The figure shows three views and two pictorial views of one solid part (mm, origin at its lowest corner). Answer the questions. Round coordinates to 2 decimals unless told otherwise and drop trailing zeros. Order: outer loops, then holes, each group sorted by start corner. A loop starts at its lowest first (then second) coordinate and runs counter-clockwise, first axis right, second up. Notation, with made-up numbers: (82.5, 25.25) -> (94.5, 25.25) arc R25 cw to (94.5, 41.25) -> close; hole circle Ø6 at (72.5, 61.5). An arc over 180 degrees is marked (long way). One line per item, written item: value. Start each with the question number.
1. Section D-D (x = 5.75) is taken. Give the vertices of the cut face in (y, z).
2. Consider line 1 (Z direction, x = 15, y = 1.35); line 2 (Z direction, x = 18, y = 0.3); line 3 (X direction, y = 0.4, z = 23). Determine where each line is inside the solid, lowest interval first.
3. Section C-C (z = 6.5) is taken. Give the vertices of the cut face in (x, y), then the cut area to 3 significant figures.
4. Section B-B (y = 0.65) is taken. Give the vertices of the cut face in (x, z).
5. Section A-A (x = 15) is taken. Give the vertices of the cut face in (y, z).
6. The mould has two halves that part along Z. Classify the marked faces 1, 2 and 3: released by +Z, released by -Z, zero draft, split by the parting line, or undercut.
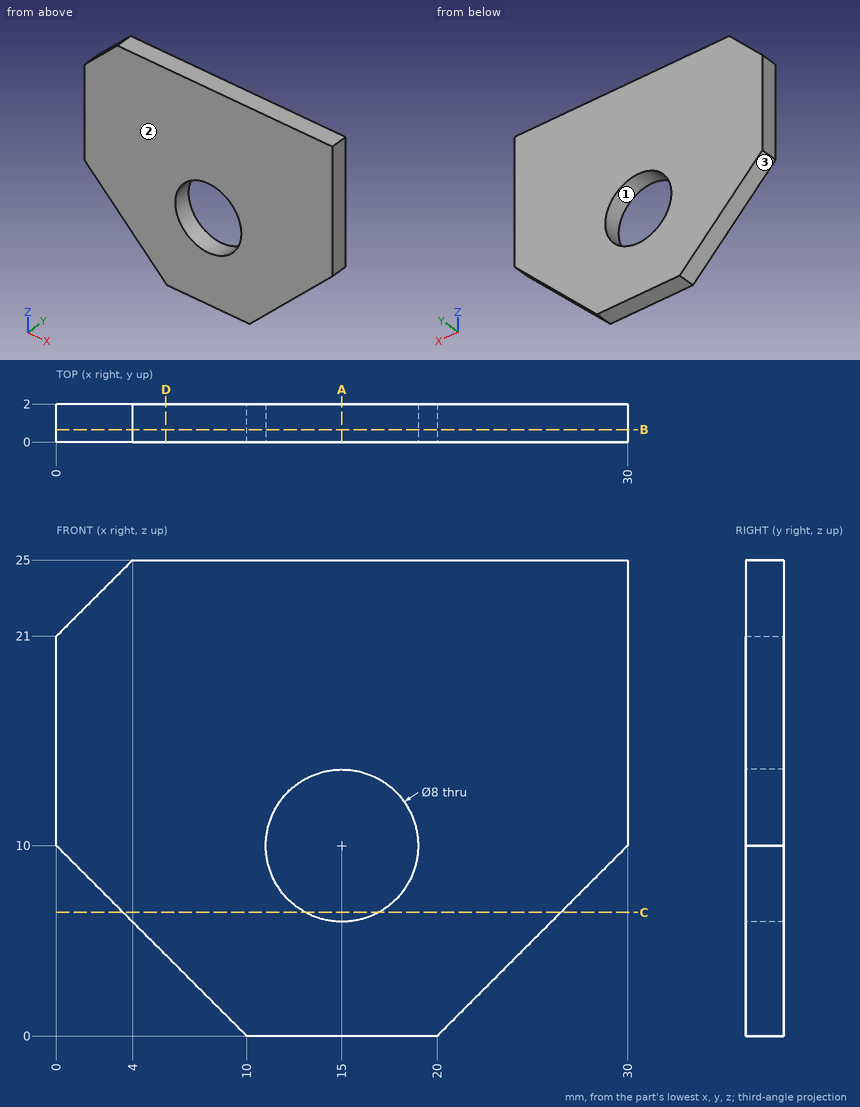
Answer:
1. outline: (0, 4.25) -> (2, 4.25) -> (2, 25) -> (0, 25) -> close
2. line 1: 0 to 6, 14 to 25
2. line 2: 0 to 7.35, 12.65 to 25
2. line 3: 2 to 30
3. outline: (3.5, 0) -> (13.06, 0) -> (13.06, 2) -> (3.5, 2) -> close; (16.94, 0) -> (26.5, 0) -> (26.5, 2) -> (16.94, 2) -> close
3. area: 38.3 mm^2
4. outline: (0, 10) -> (10, 0) -> (20, 0) -> (30, 10) -> (30, 25) -> (4, 25) -> (0, 21) -> close; hole circle Ø8 at (15, 10)
5. outline: (0, 0) -> (2, 0) -> (2, 6) -> (0, 6) -> close; (0, 14) -> (2, 14) -> (2, 25) -> (0, 25) -> close
6. face 1: undercut
6. face 2: zero draft
6. face 3: released by -Z
